```python
from build123d import *

# Parameters (mm, degrees)
SKETCH_1_R               = 49.99999999999999
EXTRUDE_1_DEPTH          = 50
CUT_EXTRUDE_2_DEPTH      = 87.60254037844385
CUT_EXTRUDE_3_DEPTH      = 76.00000000000004
FILLET_1_R               = 2
CHAMFER_1_SIZE           = 0.6
SHELL_1_T                = -1.2
EXTRUDE_2_DEPTH          = 2
EXTRUDE_2_DEPTH_BACK     = 2
SKETCH_4_R               = 1.500000000000004
SKETCH_5_R               = 1.500000000000004
EXTRUDE_3_DEPTH          = 3
CUT_EXTRUDE_4_DEPTH      = 75.75240590513992
CUT_EXTRUDE_4_DEPTH_BACK = 75.75240590513992
SKETCH_7_W               = 4
SKETCH_7_H               = 3.000000000000007
EXTRUDE_4_DEPTH          = 3
SKETCH_8_W               = 61.68253403520822
SKETCH_8_H               = 49.35584928772633
CUT_EXTRUDE_5_DEPTH      = 75.75240590513992
SKETCH_9_W               = 4
SKETCH_9_H               = 3.000000000000007
EXTRUDE_5_DEPTH          = 6.2
CHAMFER_2_SIZE           = 0.4
CHAMFER_3_SIZE           = 0.4
CHAMFER_4_SIZE           = 0.4


with BuildPart() as part:
    # 草图1 → 凸台-拉伸1 (new body)
    with BuildSketch(Plane(origin=(0, 0, 0), x_dir=(1, 0, 0), z_dir=(0, 1, 0))):
        with Locations(Location((0, 0, 0), (0, 0, 270))):
            Circle(SKETCH_1_R)
    extrude(amount=EXTRUDE_1_DEPTH)

    # 草图2 → 切除-拉伸2 (cut, through all)
    with BuildSketch(Plane(origin=(0, 50, 0), x_dir=(1, 0, 0), z_dir=(0, 1, 0))):
        with BuildLine():
            Line((-24.999999999999993, -43.301270189221945), (-7.11e-15, -1.421e-14))
            Line((7.11e-15, -1.421e-14), (25.00000000000002, -43.301270189221924))
            ThreePointArc((25.00000000000002, -43.301270189221924), (2.487e-14, 50), (-25.000000000000053, -43.30127018922191))
        make_face()
    extrude(amount=-CUT_EXTRUDE_2_DEPTH, mode=Mode.SUBTRACT)

    # 草图3 → 切除-拉伸3 (cut, through all)
    with BuildSketch(Plane(origin=(0, 50, 0), x_dir=(1, 0, 0), z_dir=(0, 1, 0))):
        with BuildLine():
            ThreePointArc((-7.5000000000002185, -12.990381056766447), (-3.882285676537599, -14.488887394336077), (6.9403e-13, -14.999999999999996))
            ThreePointArc((6.9403e-13, -14.999999999999996), (3.8822856765382965, -14.488887394335892), (7.500000000000258, -12.990381056766429))
            Line((7.5, -12.990381056766573), (0, 0))
            Line((4.01e-15, 0), (-7.499999999999988, -12.990381056766578))
        make_face()
        with BuildLine():
            ThreePointArc((15, 0), (-7.499999999999881, 12.99038105676664), (-7.5000000000002185, -12.990381056766447))
            Line((-7.499999999999988, -12.990381056766578), (4.01e-15, 0))
            Line((0, 0), (7.5, -12.990381056766573))
            ThreePointArc((7.500000000000258, -12.990381056766429), (12.99038105676665, -7.499999999999878), (15, -3.67e-15))
        make_face()
        with BuildLine():
            ThreePointArc((7.500000000000258, -12.990381056766429), (3.8822856765382965, -14.488887394335892), (6.9403e-13, -14.999999999999996))
            Line((6.9456e-13, -15), (8.660254037844409, -15))
            Line((8.660254037844393, -15.000000000000004), (7.5, -12.990381056766573))
        make_face()
        with BuildLine():
            Line((-7.499999999999988, -12.990381056766578), (-8.660254037844377, -15.000000000000002))
            Line((-8.660254037844384, -15), (6.9456e-13, -15))
            ThreePointArc((6.9403e-13, -14.999999999999996), (-3.882285676537599, -14.488887394336077), (-7.5000000000002185, -12.990381056766447))
        make_face()
    extrude(amount=-CUT_EXTRUDE_3_DEPTH, mode=Mode.SUBTRACT)

    # 圆角1
    fillet_1_edges = [part.edges().sort_by_distance(p)[0] for p in [
        (25.00000000000002, 25, 43.301270189221924),
        (-25.00000000000002, 25, 43.301270189221924),
        (-8.66025403784438, 25, 15),
        (8.6602540378444, 25, 15.000000000000002),
    ]]
    fillet(fillet_1_edges, radius=FILLET_1_R)

    # 倒角1
    chamfer_1_edges = [part.edges().sort_by_distance(p)[0] for p in [
        (8.79e-15, 0, 15),
        (-16.608380961798794, -7.11e-15, 28.766559657295183),
        (16.60838096179882, 0, 28.766559657295183),
        (2.132e-14, 0, 50),
        (8.505553499465146, 0, 15.267949192431121),
        (24.16775252630995, 0, 43.09090065934718),
        (-24.16775252630992, 0, 43.09090065934719),
        (-8.505553499465128, 0, 15.267949192431121),
    ]]
    chamfer(chamfer_1_edges, length=CHAMFER_1_SIZE)

    # 抽壳1
    shell_1_openings = [part.faces().sort_by_distance(p)[0] for p in [
        (0, 50, 34.229276229),
    ]]
    offset(amount=SHELL_1_T, openings=shell_1_openings)

    # 草图4 → 凸台-拉伸2 (add, two sides: drawn at the far end of the back side and taken through both)
    with BuildSketch(Plane(origin=(0, 0, 0), x_dir=(0, 0, -1), z_dir=(1, 0, 0)).offset(-EXTRUDE_2_DEPTH_BACK)):
        with BuildLine():
            Line((-44.5, 0), (-44.5, -3))
            ThreePointArc((-44.50000000000001, -3), (-43, -1.499999999999996), (-41.49999999999999, -3))
            Line((-41.49999999999999, -3), (-41.49999999999999, 0))
            Line((-41.49999999999999, 0), (-44.5, 0))
        make_face()
        with Locations((-43, -3)):
            Circle(SKETCH_4_R)
    extrude(amount=EXTRUDE_2_DEPTH + EXTRUDE_2_DEPTH_BACK)

    # 草图5 → 凸台-拉伸3 (add)
    with BuildSketch(Plane(origin=(2, 0, 0), x_dir=(0, 0, -1), z_dir=(1, 0, 0))):
        with Locations((-43, -3)):
            Circle(SKETCH_5_R)
    extrude_3 = extrude(amount=EXTRUDE_3_DEPTH)

    # 镜向1: 凸台-拉伸3 across plane
    add(extrude_3.mirror(Plane(origin=(0, 0, 0), x_dir=(0, 0, 1), z_dir=(1, 0, 0))))

    # 草图6 → 切除-拉伸4 (cut, two sides: drawn at the far end of the back side and taken through both)
    with BuildSketch(Plane(origin=(0, 0, 0), x_dir=(0, 0, -1), z_dir=(1, 0, 0)).offset(-CUT_EXTRUDE_4_DEPTH_BACK)):
        with BuildLine():
            ThreePointArc((-41.533119314589705, 49.97969668707788), (-27.73588672288851, 47.754377602956666), (-15.000000000000043, 42.000000000000036))
            Line((-15, 42.00000000000006), (-15, 50))
            Line((-15, 50), (-16, 50))
            Line((-16, 50), (-41.53311931459036, 50))
            Line((-41.53311931459036, 50), (-41.53311931459036, 49.97969668707786))
        make_face()
    extrude(amount=CUT_EXTRUDE_4_DEPTH + CUT_EXTRUDE_4_DEPTH_BACK, mode=Mode.SUBTRACT)

    # 草图7 → 凸台-拉伸4 (add)
    with BuildSketch(Plane(origin=(0, 1.2, 0), x_dir=(1, 0, 0), z_dir=(0, 1, 0))):
        Polygon((-3.1999999999999997, -40.3), (3.1999999999999997, -40.3), (3.2000000000000006, -45.699999999999996), (-3.199999999999999, -45.699999999999996), align=None)
        with Locations((0, -43)):
            Rectangle(SKETCH_7_W, SKETCH_7_H, mode=Mode.SUBTRACT)
    extrude(amount=EXTRUDE_4_DEPTH)

    # 草图8 → 切除-拉伸5 (cut, through all)
    with BuildSketch(Plane.XZ):
        with Locations((0.9928928322647028, 29.450924327847446)):
            Rectangle(SKETCH_8_W, SKETCH_8_H)
    extrude(amount=-CUT_EXTRUDE_5_DEPTH, mode=Mode.SUBTRACT)

    # 草图9 → 凸台-拉伸5 (add)
    with BuildSketch(Plane(origin=(0, 0, 0), x_dir=(1, 0, 0), z_dir=(0, 1, 0))):
        with Locations((0, -43)):
            Rectangle(SKETCH_9_W, SKETCH_9_H)
    extrude(amount=EXTRUDE_5_DEPTH)

    # 倒角2
    # the kernel refuses this chamfer: 0.4 mm, written as the material it takes off along each edge
    with BuildSketch(Plane(origin=(2, 0, 44.5), x_dir=(-0.999621916911297, 0, 0.027495876610578732), z_dir=(0, 1, 0))) as chamfer_2_piece_1:
        Polygon((CHAMFER_2_SIZE * 0.999621916911, -CHAMFER_2_SIZE * 0.0274958766106), (-CHAMFER_2_SIZE * 0.0274958766106, -CHAMFER_2_SIZE * 0.999621916911), (0, 0), align=None)
    extrude(amount=7.228673195186364, mode=Mode.SUBTRACT)
    with BuildSketch(Plane(origin=(-2, 0, 41.49999999999999), x_dir=(-0.027495876610586577, 0, 0.9996219169112966), z_dir=(0, 1, 0))) as chamfer_2_piece_2:
        Polygon((CHAMFER_2_SIZE * 0.999621916911, CHAMFER_2_SIZE * 0.0274958766106), (-CHAMFER_2_SIZE * 0.0274958766106, CHAMFER_2_SIZE * 0.999621916911), (0, 0), align=None)
    extrude(amount=7.228673195186364, mode=Mode.SUBTRACT)
    with BuildSketch(Plane(origin=(-2, 0, 44.5), x_dir=(-0.027495876610586577, 0, -0.9996219169112966), z_dir=(0, 1, 0))) as chamfer_2_piece_3:
        Polygon((CHAMFER_2_SIZE * 0.999621916911, -CHAMFER_2_SIZE * 0.0274958766106), (-CHAMFER_2_SIZE * 0.0274958766106, -CHAMFER_2_SIZE * 0.999621916911), (0, 0), align=None)
    extrude(amount=7.228673195186364, mode=Mode.SUBTRACT)
    with BuildSketch(Plane(origin=(2, 0, 41.49999999999999), x_dir=(-0.999621916911297, 0, -0.027495876610578732), z_dir=(0, 1, 0))) as chamfer_2_piece_4:
        Polygon((CHAMFER_2_SIZE * 0.999621916911, CHAMFER_2_SIZE * 0.0274958766106), (-CHAMFER_2_SIZE * 0.0274958766106, CHAMFER_2_SIZE * 0.999621916911), (0, 0), align=None)
    extrude(amount=7.228673195186364, mode=Mode.SUBTRACT)
    with BuildSketch(Plane(origin=(2, -4.0286731951863635, 41.49999999999999), x_dir=(-0.999621916911297, 0, -0.027495876610578732), z_dir=(0, 1, 0))) as chamfer_2_piece_5_section:
        Polygon((CHAMFER_2_SIZE * 0.999621916911, CHAMFER_2_SIZE * 0.0274958766106), (-CHAMFER_2_SIZE * 0.0274958766106, CHAMFER_2_SIZE * 0.999621916911), (0, 0), align=None)
    chamfer_2_piece_5 = extrude(amount=4.0286731951863635, mode=Mode.PRIVATE)
    chamfer_2_piece_5 = chamfer_2_piece_5 - Plane(origin=(1.8624054064801094, -3, 43), x_dir=(0, 0, -1), z_dir=(-1, 0, 0)) * Cylinder(1.500000000000004, 10, mode=Mode.PRIVATE)
    add(chamfer_2_piece_5, mode=Mode.SUBTRACT)
    with BuildSketch(Plane(origin=(-2, 0, 44.5), x_dir=(-0.027495876610586577, 0, -0.9996219169112966), z_dir=(0, -1, 0))) as chamfer_2_piece_6_section:
        Polygon((CHAMFER_2_SIZE * 0.999621916911, CHAMFER_2_SIZE * 0.0274958766106), (-CHAMFER_2_SIZE * 0.0274958766106, CHAMFER_2_SIZE * 0.999621916911), (0, 0), align=None)
    chamfer_2_piece_6 = extrude(amount=4.028673195186364, mode=Mode.PRIVATE)
    chamfer_2_piece_6 = chamfer_2_piece_6 - Plane(origin=(-1.8624054062772368, -3, 43), x_dir=(0, 0, -1), z_dir=(1, 0, 0)) * Cylinder(1.500000000000004, 10, mode=Mode.PRIVATE)
    add(chamfer_2_piece_6, mode=Mode.SUBTRACT)
    with BuildSketch(Plane(origin=(-2, -4.0286731951863635, 41.49999999999999), x_dir=(-0.027495876610586577, 0, 0.9996219169112966), z_dir=(0, 1, 0))) as chamfer_2_piece_7_section:
        Polygon((CHAMFER_2_SIZE * 0.999621916911, CHAMFER_2_SIZE * 0.0274958766106), (-CHAMFER_2_SIZE * 0.0274958766106, CHAMFER_2_SIZE * 0.999621916911), (0, 0), align=None)
    chamfer_2_piece_7 = extrude(amount=4.0286731951863635, mode=Mode.PRIVATE)
    chamfer_2_piece_7 = chamfer_2_piece_7 - Plane(origin=(-1.8624054064801103, -3, 43), x_dir=(0, 0, -1), z_dir=(1, 0, 0)) * Cylinder(1.500000000000004, 10, mode=Mode.PRIVATE)
    add(chamfer_2_piece_7, mode=Mode.SUBTRACT)
    with BuildSketch(Plane(origin=(2, 0, 44.5), x_dir=(-0.999621916911297, 0, 0.027495876610578732), z_dir=(0, -1, 0))) as chamfer_2_piece_8_section:
        Polygon((CHAMFER_2_SIZE * 0.999621916911, CHAMFER_2_SIZE * 0.0274958766106), (-CHAMFER_2_SIZE * 0.0274958766106, CHAMFER_2_SIZE * 0.999621916911), (0, 0), align=None)
    chamfer_2_piece_8 = extrude(amount=4.028673195186364, mode=Mode.PRIVATE)
    chamfer_2_piece_8 = chamfer_2_piece_8 - Plane(origin=(1.8624054062774078, -3, 43), x_dir=(0, 0, -1), z_dir=(-1, 0, 0)) * Cylinder(1.500000000000004, 10, mode=Mode.PRIVATE)
    add(chamfer_2_piece_8, mode=Mode.SUBTRACT)

    # 倒角3
    chamfer_3_edges = [part.edges().sort_by_distance(p)[0] for p in [
        (0, 6.2, 44.5),
        (-2, 6.2, 43),
        (2, 6.2, 43),
        (0, 6.2, 41.49999999999999),
        (1.8000000000000584, 6.2, 41.69999999999994),
        (-1.8000000000000587, 6.2, 41.699999999999946),
        (-1.8000000000000587, 6.2, 44.300000000000054),
        (1.800000000000062, 6.2, 44.30000000000006),
    ]]
    chamfer(chamfer_3_edges, length=CHAMFER_3_SIZE)

    # 倒角4
    chamfer_4_edges = [part.edges().sort_by_distance(p)[0] for p in [
        (5, -3, 44.50000000000001),
        (-5, -3, 44.50000000000001),
    ]]
    chamfer(chamfer_4_edges, length=CHAMFER_4_SIZE)


solid = part.part
```
For this review, take the finished solid that the model builds, in its own axes (mm). Round coordinates to 2 decimals unless told otherwise and drop trailing zeros. Order: outer loops, then holes, each group sorted by start corner. A loop starts at its lowest first (then second) coordinate and runs counter-clockwise, first axis right, second up.
Q1. We need section A-A, the plane z = 43. Give the boundary of the cut face in (x, y).
Findings below:
outline: (-5, -4.1) - (-4.6, -4.5) - (4.6, -4.5) - (5, -4.1) - (5, -1.9) - (4.6, -1.5) - (2, -1.5) - (2, 5.8) - (1.6, 6.2) - (-1.6, 6.2) - (-2, 5.8) - (-2, -1.5) - (-4.6, -1.5) - (-5, -1.9) - close
Q2. Insertion check: P1, Ø1.1, axis at y = 0.5, z = 42.5, coming from the -X side; P2, Ø1, axis at y = 4.5, z = 42.5, coming from the +X side; P3, Ø2, axis at x = -4, y = -1.5, coming from the -Z side. Each pin has a flat end and moves straight along its axis. Give the tip position at first contact, or say it passes through.
Findings below:
P1: stops at x = -2
P2: stops at x = 2
P3: stops at z = 41.59
Q3. Wall thickness on line 1 (X direction, y = 0, z = 43.65); line 2 (Y direction, x = -2.5, z = 43); line 3 (Y direction, x = 4.5, z = 42.1): over which ranges is each line inside the solid? List them lowest first.
Findings below:
line 1: x = -2 to 2
line 2: y = -4.5 to -1.5
line 3: y = -4.2 to -1.8
Q4. We need section B-B, the plane y = 0.75. Give the boundary of the cut face in (x, z).
Findings below:
outline: (-2, 41.9) - (-1.6, 41.5) - (1.6, 41.5) - (2, 41.9) - (2, 44.1) - (1.6, 44.5) - (-1.6, 44.5) - (-2, 44.1) - close
Q5. We need section C-C, the plane x = 1. Give the boundary of the cut face in (y, z), plus the area to 3 significant figures.
Findings below:
outline: (-3, 41.5) - (5.8, 41.5) - (6.2, 41.9) - (6.2, 44.1) - (5.8, 44.5) - (-3, 44.5) arc R1.5 ccw to start
area: 31.0 mm2
Q6. We need section D-D, the plane x = 3. Give the boundary of the cut face in (y, z), plus the area to 3 significant figures.
Findings below:
outline: circle Ø3 at (-3, 43)
area: 7.07 mm2
